Design review of the part built by this model. Coordinates are the model's own, in mm. A direction names the side the tool comes from. Round coordinates to 2 decimals unless told otherwise and drop trailing zeros. Loops run counter-clockwise (first coordinate to the right, second up) from the corner with the lowest first, then second, coordinate; pieces in that order, holes last. Notation, with made-up numbers: (32, 44.25) - (54, 44.25) arc R20 cw to (54, 77.25) - close; hole circle Ø9 at (79, 24). An arc over 180 degrees is marked (long way). Return JSON: item names as keys, results as strings. Group by question number.
(1) Clearance check with flat-ended pins moving along their axes: pin 1 (2.5 mm diameter, centred on x = 9.7, z = 24.2, fed in from -Y); pin 2 (6 mm diameter, centred on y = 19, z = 19.5, fed in from +X); pin 3 (0.9 mm diameter, centred on x = -24.5, z = -15.5, fed in from +Y). State where each tip first meets the part, or that it passes through.
(2) We need section C-C, the plane x = -99. Write out the cut boundary in (y, z).
(3) For faces 1 (the cylindrical face through (-8.24, 11.97, -16.34)), 2 (the flat face through (-4, 14, 33)), 3 (the flat face through (0, 2.5, 0)), 4 (the flat face through (54, 6, 0)), list the 3-axis set-ups (+Z, -Z, +X, -X, +Y, -Y) from which the entire face can be reached by the end or side of a thin tool; tool diameter is ignored.
(4) We need section B-B, the plane x = 20.5. Write out the cut boundary in (y, z) (3 decimals), and give its area (3 significant figures).
(5) The part is to be moulded in two halves that separate along Z. For faces 5 (the cylindrical face through (118, 8, -57)), 6 (the flat face through (53, 4, 7.75)), 7 (the flat face through (-24, 14, -14)), say which applies: pulls with the +Z half, pulls with the -Z half, needs draft (parallel to the pull), parting line crosses it, or undercut.
(6) Wall thickness on L1, parallel to Y at x = 52, z = 19; L2, parallel to Z at x = 3.5, y = 18.5; L3, parallel to X at y = 3.5, z = 27: over which ranges is each line inside the solid? List them lowest first. Write a range as [from, to].
(7) We need section A-A, the plane y = 18.75. Write out the cut boundary in (x, z), and give its area (3 significant figures).
from build123d import *

# Parameters (mm, degrees)
SKETCH1_W                      = 240
SKETCH1_H                      = 116
BOSS_EXTRUDE1_DEPTH            = 10
SKETCH2_W                      = 62.15
SKETCH2_H                      = 62.15
CUT_EXTRUDE1_DEPTH             = 2.5
CUT_EXTRUDE2_REACH             = 135.493
SKETCH3_R                      = 1.5
SKETCH4_W                      = 12
SKETCH4_H                      = 15.5
CUT_EXTRUDE3_DEPTH             = 2.5
CUT_EXTRUDE4_REACH             = 135.493
SKETCH6_R                      = 1.5
CUT_EXTRUDE4_DIRECTION_2_DEPTH = 134.492509153
CUT_EXTRUDE5_REACH             = 135.493
SKETCH7_W                      = 6
SKETCH7_H                      = 15.5
SKETCH8_R                      = 2.5
SKETCH8_R_2                    = 1.5
SKETCH8_R_3                    = 2.347298944
BOSS_EXTRUDE2_DEPTH            = 15
SKETCH9_R                      = 2.5
SKETCH9_R_2                    = 1.5
SKETCH9_W                      = 19.78
SKETCH9_H                      = 34.766
SKETCH9_W_2                    = 17.78
SKETCH9_H_2                    = 32.766
BOSS_EXTRUDE3_DEPTH            = 4
FILLET1_R                      = 5
CUT_EXTRUDE15_REACH            = 136.123
SKETCH25_R                     = 1.5


with BuildPart() as part:
    # Sketch1 → Boss-Extrude1 (new body)
    with BuildSketch(Plane(origin=(0, 0, 0), x_dir=(1, 0, 0), z_dir=(0, 1, 0))):
        Rectangle(SKETCH1_W, SKETCH1_H)
    extrude(amount=BOSS_EXTRUDE1_DEPTH)

    # Sketch2 → Cut-Extrude1 (cut)
    with BuildSketch(Plane.XZ):
        Rectangle(SKETCH2_W, SKETCH2_H)
    extrude(amount=-CUT_EXTRUDE1_DEPTH, mode=Mode.SUBTRACT)

    # Sketch3 → Cut-Extrude2 (cut, up to next)
    with BuildSketch(Plane.XZ.offset(-2.5), mode=Mode.PRIVATE) as cut_extrude2_sk1:
        with Locations(Location((-26.075, 26.075, 0), (0, 0, 270))):
            Circle(SKETCH3_R)
    cut_extrude2_tool1 = extrude(cut_extrude2_sk1.sketch, amount=-CUT_EXTRUDE2_REACH, mode=Mode.PRIVATE) & part.part
    # Sketch3 → Cut-Extrude2 (cut, up to next)
    with BuildSketch(Plane.XZ.offset(-2.5), mode=Mode.PRIVATE) as cut_extrude2_sk2:
        with Locations(Location((-26.075, -26.075, 0), (0, 0, 90))):
            Circle(SKETCH3_R)
    cut_extrude2_tool2 = extrude(cut_extrude2_sk2.sketch, amount=-CUT_EXTRUDE2_REACH, mode=Mode.PRIVATE) & part.part
    # Sketch3 → Cut-Extrude2 (cut, up to next)
    with BuildSketch(Plane.XZ.offset(-2.5), mode=Mode.PRIVATE) as cut_extrude2_sk3:
        with Locations(Location((26.075, -26.075, 0), (0, 0, 270))):
            Circle(SKETCH3_R)
    cut_extrude2_tool3 = extrude(cut_extrude2_sk3.sketch, amount=-CUT_EXTRUDE2_REACH, mode=Mode.PRIVATE) & part.part
    # Sketch3 → Cut-Extrude2 (cut, up to next)
    with BuildSketch(Plane.XZ.offset(-2.5), mode=Mode.PRIVATE) as cut_extrude2_sk4:
        with Locations(Location((26.075, 26.075, 0), (0, 0, 90))):
            Circle(SKETCH3_R)
    cut_extrude2_tool4 = extrude(cut_extrude2_sk4.sketch, amount=-CUT_EXTRUDE2_REACH, mode=Mode.PRIVATE) & part.part
    add(cut_extrude2_tool1.solids().sort_by_distance((-26.075, 2.5, 26.075))[0], mode=Mode.SUBTRACT)
    add(cut_extrude2_tool2.solids().sort_by_distance((-26.075, 2.5, -26.075))[0], mode=Mode.SUBTRACT)
    add(cut_extrude2_tool3.solids().sort_by_distance((26.075, 2.5, -26.075))[0], mode=Mode.SUBTRACT)
    add(cut_extrude2_tool4.solids().sort_by_distance((26.075, 2.5, 26.075))[0], mode=Mode.SUBTRACT)

    # Sketch4 → Cut-Extrude3 (cut)
    with BuildSketch(Plane.XZ):
        with Locations((54, 0)):
            Rectangle(SKETCH4_W, SKETCH4_H)
    extrude(amount=-CUT_EXTRUDE3_DEPTH, mode=Mode.SUBTRACT)

    # Sketch6 → Cut-Extrude4 (cut, up to next)
    with BuildSketch(Plane.XZ.offset(-2.5), mode=Mode.PRIVATE) as cut_extrude4_sk1:
        with Locations(Location((58, 5.75, 0), (0, 0, 90))):
            Circle(SKETCH6_R)
    cut_extrude4_tool1 = extrude(cut_extrude4_sk1.sketch, amount=-CUT_EXTRUDE4_REACH, mode=Mode.PRIVATE) & part.part
    # Sketch6 → Cut-Extrude4 (cut, up to next)
    with BuildSketch(Plane.XZ.offset(-2.5), mode=Mode.PRIVATE) as cut_extrude4_sk2:
        with Locations(Location((58, -5.75, 0), (0, 0, 90))):
            Circle(SKETCH6_R)
    cut_extrude4_tool2 = extrude(cut_extrude4_sk2.sketch, amount=-CUT_EXTRUDE4_REACH, mode=Mode.PRIVATE) & part.part
    add(cut_extrude4_tool1.solids().sort_by_distance((58, 2.5, 5.75))[0], mode=Mode.SUBTRACT)
    add(cut_extrude4_tool2.solids().sort_by_distance((58, 2.5, -5.75))[0], mode=Mode.SUBTRACT)

    # Sketch6 → Cut-Extrude4 direction 2 (cut)
    with BuildSketch(Plane.XZ.offset(-2.5)):
        with Locations(Location((58, 5.75, 0), (0, 0, 90))):
            Circle(SKETCH6_R)
        with Locations(Location((58, -5.75, 0), (0, 0, 90))):
            Circle(SKETCH6_R)
    extrude(amount=CUT_EXTRUDE4_DIRECTION_2_DEPTH, mode=Mode.SUBTRACT)

    # Sketch7 → Cut-Extrude5 (cut, up to next)
    with BuildSketch(Plane.XZ.offset(-2.5), mode=Mode.PRIVATE) as cut_extrude5_sk1:
        with Locations((51, 0)):
            Rectangle(SKETCH7_W, SKETCH7_H)
    cut_extrude5_tool1 = extrude(cut_extrude5_sk1.sketch, amount=-CUT_EXTRUDE5_REACH, mode=Mode.PRIVATE) & part.part
    add(cut_extrude5_tool1.solids().sort_by_distance((51, 2.5, 0))[0], mode=Mode.SUBTRACT)

    # Sketch8 → Boss-Extrude2 (add)
    # profile 1 of 4: a face of its own
    with BuildSketch(Plane(origin=(0, 10, 0), x_dir=(1, 0, 0), z_dir=(0, 1, 0))):
        with Locations(Location((86.5, 24.2, 0), (0, 0, 270))):
            Circle(SKETCH8_R)
        with Locations(Location((86.5, 24.2, 0), (0, 0, 270))):
            Circle(SKETCH8_R_2, mode=Mode.SUBTRACT)
    # profile 2 of 4: a face of its own
    with BuildSketch(Plane(origin=(0, 10, 0), x_dir=(1, 0, 0), z_dir=(0, 1, 0))):
        with Locations(Location((84.5, -24.2, 0), (0, 0, 270))):
            Circle(SKETCH8_R_3)
        with Locations(Location((84.5, -24.2, 0), (0, 0, 270))):
            Circle(SKETCH8_R_2, mode=Mode.SUBTRACT)
    # profile 3 of 4: a face of its own
    with BuildSketch(Plane(origin=(0, 10, 0), x_dir=(1, 0, 0), z_dir=(0, 1, 0))):
        with Locations(Location((9.7, -24.2, 0), (0, 0, 270))):
            Circle(SKETCH8_R)
        with Locations(Location((9.7, -24.2, 0), (0, 0, 270))):
            Circle(SKETCH8_R_2, mode=Mode.SUBTRACT)
    # profile 4 of 4: a face of its own
    with BuildSketch(Plane(origin=(0, 10, 0), x_dir=(1, 0, 0), z_dir=(0, 1, 0))):
        with Locations(Location((2.7, 24.2, 0), (0, 0, 270))):
            Circle(SKETCH8_R)
        with Locations(Location((2.7, 24.2, 0), (0, 0, 270))):
            Circle(SKETCH8_R_2, mode=Mode.SUBTRACT)
    extrude(amount=BOSS_EXTRUDE2_DEPTH)

    # Sketch9 → Boss-Extrude3 (add)
    # profile 1 of 6: a face of its own
    with BuildSketch(Plane(origin=(0, 10, 0), x_dir=(1, 0, 0), z_dir=(0, 1, 0))):
        with Locations(Location((-24.1, 15.8, 0), (0, 0, 270))):
            Circle(SKETCH9_R)
        with Locations(Location((-24.1, 15.8, 0), (0, 0, 270))):
            Circle(SKETCH9_R_2, mode=Mode.SUBTRACT)
    # profile 2 of 6: a face of its own
    with BuildSketch(Plane(origin=(0, 10, 0), x_dir=(1, 0, 0), z_dir=(0, 1, 0))):
        with Locations(Location((-5.8, 15.8, 0), (0, 0, 270))):
            Circle(SKETCH9_R)
        with Locations(Location((-5.8, 15.8, 0), (0, 0, 270))):
            Circle(SKETCH9_R_2, mode=Mode.SUBTRACT)
    # profile 3 of 6: a face of its own
    with BuildSketch(Plane(origin=(0, 10, 0), x_dir=(1, 0, 0), z_dir=(0, 1, 0))):
        with Locations(Location((-5.8, 42.5, 0), (0, 0, 270))):
            Circle(SKETCH9_R)
        with Locations(Location((-5.8, 42.5, 0), (0, 0, 270))):
            Circle(SKETCH9_R_2, mode=Mode.SUBTRACT)
    # profile 4 of 6: a face of its own
    with BuildSketch(Plane(origin=(0, 10, 0), x_dir=(1, 0, 0), z_dir=(0, 1, 0))):
        Polygon((-17.7, -47), (-17.7, -48), (-22.7, -48), (-22.7, -22.8), (-3.3, -22.8), (-3.3, -48), (-8.3, -48), (-8.3, -47), (-4.3, -47), (-4.3, -23.8), (-21.7, -23.8), (-21.7, -47), align=None)
    # profile 5 of 6: a face of its own
    with BuildSketch(Plane(origin=(0, 10, 0), x_dir=(1, 0, 0), z_dir=(0, 1, 0))):
        Polygon((-41.1, -48), (-46.1, -48), (-46.1, -22.8), (-26.7, -22.8), (-26.7, -48), (-31.7, -48), (-31.7, -47), (-27.7, -47), (-27.7, -23.8), (-45.1, -23.8), (-45.1, -47), (-41.1, -47), align=None)
    # profile 6 of 6: a face of its own
    with BuildSketch(Plane(origin=(0, 10, 0), x_dir=(1, 0, 0), z_dir=(0, 1, 0))):
        with Locations((-41.35, 26)):
            Rectangle(SKETCH9_W, SKETCH9_H)
        with Locations((-41.35, 26)):
            Rectangle(SKETCH9_W_2, SKETCH9_H_2, mode=Mode.SUBTRACT)
    extrude(amount=BOSS_EXTRUDE3_DEPTH)

    # Fillet1
    fillet1_edges = [part.edges().sort_by_distance(p)[0] for p in [
        (0, 0, 58),
        (-120, 0, 0),
        (0, 0, -58),
        (120, 0, 0),
        (120, 5, 58),
        (-120, 5, 58),
        (-120, 5, -58),
        (120, 5, -58),
    ]]
    fillet(fillet1_edges, radius=FILLET1_R)

    # Sketch25 → Cut-Extrude15 (cut, up to next)
    with BuildSketch(Plane(origin=(0, 10, 0), x_dir=(1, 0, 0), z_dir=(0, 1, 0)), mode=Mode.PRIVATE) as cut_extrude15_sk1:
        with Locations(Location((-115, 53, 0), (0, 0, 270))):
            Circle(SKETCH25_R)
    cut_extrude15_tool1 = extrude(cut_extrude15_sk1.sketch, amount=-CUT_EXTRUDE15_REACH, mode=Mode.PRIVATE) & part.part
    # Sketch25 → Cut-Extrude15 (cut, up to next)
    with BuildSketch(Plane(origin=(0, 10, 0), x_dir=(1, 0, 0), z_dir=(0, 1, 0)), mode=Mode.PRIVATE) as cut_extrude15_sk2:
        with Locations(Location((-115, -53, 0), (0, 0, 270))):
            Circle(SKETCH25_R)
    cut_extrude15_tool2 = extrude(cut_extrude15_sk2.sketch, amount=-CUT_EXTRUDE15_REACH, mode=Mode.PRIVATE) & part.part
    # Sketch25 → Cut-Extrude15 (cut, up to next)
    with BuildSketch(Plane(origin=(0, 10, 0), x_dir=(1, 0, 0), z_dir=(0, 1, 0)), mode=Mode.PRIVATE) as cut_extrude15_sk3:
        with Locations(Location((115, -53, 0), (0, 0, 270))):
            Circle(SKETCH25_R)
    cut_extrude15_tool3 = extrude(cut_extrude15_sk3.sketch, amount=-CUT_EXTRUDE15_REACH, mode=Mode.PRIVATE) & part.part
    # Sketch25 → Cut-Extrude15 (cut, up to next)
    with BuildSketch(Plane(origin=(0, 10, 0), x_dir=(1, 0, 0), z_dir=(0, 1, 0)), mode=Mode.PRIVATE) as cut_extrude15_sk4:
        with Locations(Location((115, 53, 0), (0, 0, 270))):
            Circle(SKETCH25_R)
    cut_extrude15_tool4 = extrude(cut_extrude15_sk4.sketch, amount=-CUT_EXTRUDE15_REACH, mode=Mode.PRIVATE) & part.part
    add(cut_extrude15_tool1.solids().sort_by_distance((-115, 10, -53))[0], mode=Mode.SUBTRACT)
    add(cut_extrude15_tool2.solids().sort_by_distance((-115, 10, 53))[0], mode=Mode.SUBTRACT)
    add(cut_extrude15_tool3.solids().sort_by_distance((115, 10, 53))[0], mode=Mode.SUBTRACT)
    add(cut_extrude15_tool4.solids().sort_by_distance((115, 10, -53))[0], mode=Mode.SUBTRACT)


solid = part.part
Solutions:
{
 "1": {"pin 1": "y = 2.5", "pin 2": "x = 86.12", "pin 3": "y = 10"},
 "2": {"outline": "(0, -53) arc R5 ccw to (5, -58) - (10, -58) - (10, 58) - (5, 58) arc R5 ccw to (0, 53) - close"},
 "3": {"face 1": "+Y", "face 2": "+Z, -Z, -X, +Y", "face 3": "-Y", "face 4": "+Y, -Y"},
 "4": {"outline": "(0, -53) arc R5 ccw to (5, -58) - (10, -58) - (10, 58) - (5, 58) arc R5 ccw to (0, 53) - (0, 31.075) - (2.5, 31.075) - (2.5, -31.075) - (0, -31.075) - close", "area": "994 mm^2"},
 "5": {"face 5": "pulls with the -Z half", "face 6": "undercut", "face 7": "needs draft"},
 "6": {"L1": "[0, 10]", "L2": "[-26.57, -25.47], [-22.93, -21.83]", "L3": "[-119.77, -27.26], [-24.89, 24.89], [27.26, 119.77]"},
 "7": {"outline": "circle Ø5 at (2.7, -24.2); circle Ø5 at (9.7, 24.2); circle Ø4.69 at (84.5, 24.2); circle Ø5 at (86.5, -24.2); hole circle Ø3 at (2.7, -24.2); hole circle Ø3 at (9.7, 24.2); hole circle Ø3 at (84.5, 24.2); hole circle Ø3 at (86.5, -24.2)", "area": "47.9 mm^2"}
}
